```python
from build123d import *

# Parameters (mm, degrees)
BOSS_EXTRUDE1_DEPTH     = 3.75
CUT_EXTRUDE1_DEPTH      = 48.166697998
CUT_EXTRUDE1_DEPTH_BACK = 48.166697998
SKETCH2_R               = 1.5
BOSS_EXTRUDE2_START     = -4
SKETCH3_R               = 3.75
BOSS_EXTRUDE2_DEPTH     = 29
SKETCH4_R               = 3
SKETCH4_R_2             = 3.75
BOSS_EXTRUDE3_DEPTH     = 3
CUT_EXTRUDE2_DEPTH      = 1


with BuildPart() as part:
    # Sketch1 → Boss-Extrude1 (new, symmetric)
    with BuildSketch(Plane(origin=(0, 0, 0), x_dir=(-1, 0, 0), z_dir=(0, 1, 0))):
        with BuildLine():
            Line((-36.93, 2.1), (-28.70870948, 2.1))
            ThreePointArc((-28.70870948, 2.1), (-27.398273911, 2.589119918), (-26.728798481, 3.817241379))
            ThreePointArc((-26.728798481, 3.817241379), (0.047012438, 26.999959071), (26.741929561, 3.724137931))
            ThreePointArc((26.741929561, 3.724137931), (27.409748904, 2.491403941), (28.722813233, 2))
            Line((28.722813233, 2), (33.18, 2))
            Line((33.18, 2), (33.18, -2))
            Line((33.18, -2), (28.722813233, -2))
            ThreePointArc((28.722813233, -2), (27.409748904, -2.491403941), (26.741929561, -3.724137931))
            ThreePointArc((26.741929561, -3.724137931), (0.047012438, -26.999959071), (-26.728798481, -3.817241379))
            ThreePointArc((-26.728798481, -3.817241379), (-27.398273911, -2.589119918), (-28.70870948, -2.1))
            Line((-28.70870948, -2.1), (-36.93, -2.1))
            Line((-36.93, -2.1), (-36.93, -0.2))
            Line((-36.93, -0.2), (-24.999199987, -0.2))
            ThreePointArc((-24.999199987, -0.2), (25, 0), (-24.999199987, 0.2))
            Line((-24.999199987, 0.2), (-36.93, 0.2))
            Line((-36.93, 0.2), (-36.93, 2.1))
        make_face()
    extrude(amount=BOSS_EXTRUDE1_DEPTH, both=True)

    # Sketch2 → Cut-Extrude1 (cut, two sides: drawn at the far end of the back side and taken through both)
    with BuildSketch(Plane.XY.offset(2.1).offset(-CUT_EXTRUDE1_DEPTH_BACK)):
        with BuildLine():
            Line((36.93, 0), (36.93, 3.75))
            Line((36.93, 3.75), (33.18, 3.75))
            ThreePointArc((33.18, 3.75), (35.831650429, 2.651650429), (36.93, 0))
        make_face()
        with BuildLine():
            Line((36.93, -3.75), (36.93, 0))
            ThreePointArc((36.93, 0), (35.831650429, -2.651650429), (33.18, -3.75))
            Line((33.18, -3.75), (36.93, -3.75))
        make_face()
        with Locations((33.18, 0)):
            Circle(SKETCH2_R)
    extrude(amount=CUT_EXTRUDE1_DEPTH + CUT_EXTRUDE1_DEPTH_BACK, mode=Mode.SUBTRACT)

    # Sketch3 → Boss-Extrude2 (add)
    with BuildSketch(Plane.XY.offset(2).offset(BOSS_EXTRUDE2_START)):
        with Locations(Location((-33.17, 0, 0), (0, 0, 180))):
            Circle(SKETCH3_R)
    extrude(amount=BOSS_EXTRUDE2_DEPTH)


with BuildPart() as body_2:
    # Body-Move/Copy1: copy of part
    add(part.part.moved(Location((0, -72.5, 0))))


with BuildPart() as part_1:
    add(part.part)

    add(body_2.part)  # Boss-Extrude3 merges body 2
    # Sketch4 → Boss-Extrude3 (add)
    # profile 1 of 2: a face of its own
    with BuildSketch(Plane.XY.offset(27)):
        with BuildLine():
            ThreePointArc((-63.482977809, -51.870117717), (-48.248375933, -60.895538839), (-37.114961483, -74.665012447))
            ThreePointArc((-37.114961483, -74.665012447), (-31.545330888, -76.696480701), (-28.795616265, -71.444174757))
            ThreePointArc((-28.795616265, -71.444174757), (-32.982825115, -36.25), (-28.795616265, -1.055825243))
            ThreePointArc((-28.795616265, -1.055825243), (-31.524893516, 4.188511031), (-37.09366658, 2.203370275))
            ThreePointArc((-37.09366658, 2.203370275), (-50.421900488, -17.640799048), (-66.733284536, -35.115684618))
            ThreePointArc((-66.733284536, -35.115684618), (-69.806976307, -44.404462177), (-63.482977809, -51.870117717))
        make_face()
        with Locations((-59.99, -42.5)):
            Circle(SKETCH4_R, mode=Mode.SUBTRACT)
        with Locations(Location((-33.17, -72.5, 0), (0, 0, 180))):
            Circle(SKETCH4_R_2, mode=Mode.SUBTRACT)
    # profile 2 of 2: a face of its own
    with BuildSketch(Plane.XY.offset(27)):
        with Locations(Location((-33.17, -72.5, 0), (0, 0, 180))):
            Circle(SKETCH4_R_2)
    extrude(amount=BOSS_EXTRUDE3_DEPTH)

    # Sketch5 → Cut-Extrude2 (cut)
    with BuildSketch(Plane(origin=(0, 0, 27), x_dir=(1, 0, 0), z_dir=(0, 0, -1))):
        with BuildLine():
            Line((-38.884156213, 63.752554506), (-36.884156213, 63.752554506))
            ThreePointArc((-36.884156213, 63.752554506), (-35.358719938, 63.046016594), (-34.911062224, 61.425598679))
            ThreePointArc((-34.911062224, 61.425598679), (-36.978469514, 35.091765908), (-34.515193771, 8.792009371))
            ThreePointArc((-34.515193771, 8.792009371), (-35.751988173, 6.573851631), (-38.16775438, 7.357406215))
            ThreePointArc((-38.16775438, 7.357406215), (-48.567697695, 21.716067782), (-60.549030633, 34.784259851))
            ThreePointArc((-60.549030633, 34.784259851), (-60.782300133, 35.868309862), (-59.871765467, 36.501165064))
            ThreePointArc((-59.871765467, 36.501165064), (-54.085301002, 41.434856938), (-57.783175082, 48.079419663))
            ThreePointArc((-57.783175082, 48.079419663), (-58.414835004, 48.976588199), (-57.843234491, 49.913166275))
            ThreePointArc((-57.843234491, 49.913166275), (-48.441923829, 55.600366923), (-40.386431593, 63.072845642))
            ThreePointArc((-40.386431593, 63.072845642), (-39.708600792, 63.574721111), (-38.884156213, 63.752554506))
        make_face()
    extrude(amount=-CUT_EXTRUDE2_DEPTH, mode=Mode.SUBTRACT)


solid = part_1.part
```
Can you work these out from the model? Positions are in its coordinate system, mm. A direction names the side the tool comes from. Coordinates: 2 decimals unless noted, no trailing zeros. Order: outer loops, then holes, each group sorted by start corner. A loop starts at its lowest first (then second) coordinate and runs counter-clockwise, first axis right, second up.
1. Thinking about a two-plate mould opening in Y: for faces 4 (the face through (-69.833, -44.264, 28.479)), 5 (the face through (-33, -73, -2)), 6 (the face through (-25, -68.75, -4)), which applies, +Y half, -Y half, draft (parallel to the pull), parting line (faces both ways), or undercut?
2. For faces 1 (the face through (31, 0, -2.1)), 2 (the face through (-36.98, -35.46, 27.49)), 3 (the face through (31, -72, 2.1)), which set-ups out of +Z, -Z, +X, -X, +Y, -Y let a thin tool reach every point of the face, with its end or its side?
3. If we section it at C-C (y = -42.5): Please give me the cut outline in (x, z).
4. I'm going to push flat-ended pins straight in: pin 1 (2.5 mm diameter, centred on x = 31.5, y = -1, fed in from +Z); pin 2 (12 mm diameter, centred on y = -34, z = 22, fed in from -X); pin 3 (5 mm diameter, centred on x = -46.5, y = -62, fed in from -Z). Where does each tip first touch, or does it pass through?
5. I need wall thicknesses on line 1 (Y direction, x = 33.18, z = -1); line 2 (Y direction, x = 33, z = -1); line 3 (Z direction, x = 0, y = 0). Which ranges of each line are inside material? Lowest first, please.
6. If we section it at D-D (z = -10): Please give me the cut outline in (x, y), then the cut area to 3 significant figures.
7. If we section it at B-B (z = 22): Please give me the cut outline in (x, y).
8. If we section it at A-A (x = 0): Please give me the cut outline in (y, z), then the cut area to 3 significant figures.
Entries:
1. face 4: parting line
1. face 5: draft
1. face 6: undercut
2. face 1: -Z, +X, +Y, -Y
2. face 2: -Z
2. face 3: +Z, +X, +Y, -Y
3. outline: (-69.99, 27) - (-62.99, 27) - (-62.99, 30) - (-69.99, 30) - close; (-56.99, 27) - (-53.99, 27) - (-53.99, 28) - (-36.86, 28) - (-36.86, 27) - (-32.85, 27) - (-32.85, 30) - (-56.99, 30) - close
4. pin 1: stops at z = 2.1
4. pin 2: stops at x = -68.54
4. pin 3: stops at z = 27
5. line 1: y = -76.25 to -74, -71 to -68.75, -3.75 to -1.5, 1.5 to 3.75
5. line 2: y = -76.25 to -73.99, -71.01 to -68.75, -3.75 to -1.49, 1.49 to 3.75
5. line 3: z = -27 to -25, 25 to 27
6. outline: (-25.08, -76.25) - (-22.91, -76.25) - (-22.91, -68.75) - (-25.08, -68.75) - close; (-25.08, -3.75) - (-22.91, -3.75) - (-22.91, 3.75) - (-25.08, 3.75) - close; (22.91, -76.25) - (25.08, -76.25) - (25.08, -68.75) - (22.91, -68.75) - close; (22.91, -3.75) - (25.08, -3.75) - (25.08, 3.75) - (22.91, 3.75) - close
6. area: 65.0 mm2
7. outline: circle Ø7.5 at (-33.17, -72.5); circle Ø7.5 at (-33.17, 0); (-15.65, -76.25) - (-11.87, -76.25) - (-11.87, -68.75) - (-15.65, -68.75) - close; (-15.65, -3.75) - (-11.87, -3.75) - (-11.87, 3.75) - (-15.65, 3.75) - close; (11.87, -76.25) - (15.65, -76.25) - (15.65, -68.75) - (11.87, -68.75) - close; (11.87, -3.75) - (15.65, -3.75) - (15.65, 3.75) - (11.87, 3.75) - close
8. outline: (-76.25, -27) - (-68.75, -27) - (-68.75, -25) - (-76.25, -25) - close; (-76.25, 25) - (-68.75, 25) - (-68.75, 27) - (-76.25, 27) - close; (-3.75, -27) - (3.75, -27) - (3.75, -25) - (-3.75, -25) - close; (-3.75, 25) - (3.75, 25) - (3.75, 27) - (-3.75, 27) - close
8. area: 60.0 mm2
